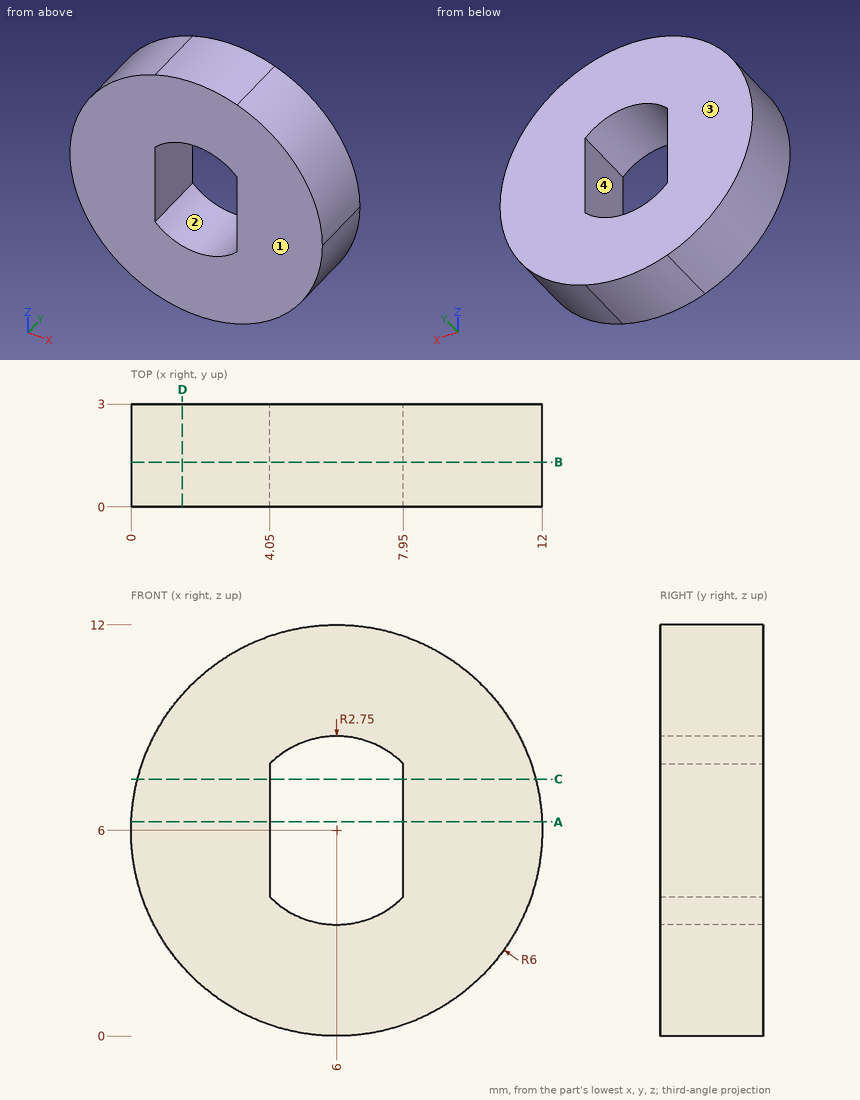
Check sheet for the drawn part. Datum: minimum x, y, z corner. Units: mm. A direction names the side the tool comes from. Round coordinates to 2 decimals unless told otherwise and drop trailing zeros. Order: outer loops, then holes, each group sorted by start corner. A loop starts at its lowest first (then second) coordinate and runs counter-clockwise, first axis right, second up. Notation, with made-up numbers: (74, 53.25) -> (118, 53.25) arc R10 cw to (118, 65.25) -> close; hole circle Ø5 at (76, 27). An arc over 180 degrees is marked (long way). Put each result on its own line as item: value. Start each with the question number.
(1) Draft check along X on the marked faces 1 and 2. Enter one of: +X half, -X half, draft (parallel to the pull), parting line (faces both ways), or undercut.
(2) Material ranges on line 1 along Z through (x, y) = (6, 0.85); line 2 along X through (y, z) = (0.65, 4.5); line 3 along Z through (x, y) = (5, 2.5), recorded low to high.
(3) Section check B-B (y = 1.3). Enter the section's corners in (x, z).
(4) Section check C-C (z = 7.5). Enter the section's corners in (x, y), then the cut area to 3 significant figures.
(5) Section check A-A (z = 6.25). Enter the section's corners in (x, y).
(6) Section check D-D (x = 1.5). Enter the section's corners in (y, z), then the cut area to 3 significant figures.
(7) Tool access check on the marked faces 3 and 4. Record the directions out of +Z, -Z, +X, -X, +Y, -Y that give a thin tool (end or side, any length) a straight path to the whole face; none if there is none.
Completed:
1. face 1: draft
1. face 2: undercut
2. line 1: z = 0 to 3.25, 8.75 to 12
2. line 2: x = 0.19 to 4.05, 7.95 to 11.81
2. line 3: z = 0.08 to 3.44, 8.56 to 11.92
3. outline: circle Ø12 at (6, 6); hole (4.05, 4.06) arc R2.75 ccw to (7.95, 4.06) -> (7.95, 7.94) arc R2.75 ccw to (4.05, 7.94) -> close
4. outline: (0.19, 0) -> (4.05, 0) -> (4.05, 3) -> (0.19, 3) -> close; (7.95, 0) -> (11.81, 0) -> (11.81, 3) -> (7.95, 3) -> close
4. area: 23.2 mm2
5. outline: (0.01, 0) -> (4.05, 0) -> (4.05, 3) -> (0.01, 3) -> close; (7.95, 0) -> (11.99, 0) -> (11.99, 3) -> (7.95, 3) -> close
6. outline: (0, 2.03) -> (3, 2.03) -> (3, 9.97) -> (0, 9.97) -> close
6. area: 23.8 mm2
7. face 3: +Z, -Z, +X, -X, +Y
7. face 4: +Y, -Y
